CAD build for the part. Positions are in the model's coordinates, mm. A direction names the side the tool comes from. Round coordinates to 2 decimals unless told otherwise and drop trailing zeros. Loops run counter-clockwise (first coordinate to the right, second up) from the corner with the lowest first, then second, coordinate; pieces in that order, holes last. Notation, with made-up numbers: M 18.25,62 L 58.25,62 A30 ccw 58.25,91 Z; hole C -15.5,85 d7. An arc over 180 degrees is marked long. One line per item, written item: value. Start each with the question number.
from build123d import *

# Parameters (mm, degrees)
BASE_FLANGE1_DEPTH   = 0.7366
FILLET1_R            = 5
FILLET2_R            = 5
FILLET3_R            = 5
FILLET4_R            = 5
EDGE_FLANGE2_START   = -47.5
EDGE_FLANGE2_DEPTH   = 15.3683
EDGE_FLANGE2_START_2 = -32.5
EDGE_FLANGE2_2_DEPTH = 0.3683
EDGE_FLANGE2_3_DEPTH = 15
FILLET7_R            = 5
FILLET8_R            = 5
SKETCH18_R           = 1.5
CUT_EXTRUDE1_DEPTH   = 40
SKETCH23_R           = 1.52
CUT_EXTRUDE6_DEPTH   = 30
SKETCH24_R           = 1.52
CUT_EXTRUDE7_DEPTH   = 30
SKETCH25_R           = 1.4
CUT_EXTRUDE8_DEPTH   = 10


with BuildPart() as part:
    # Base-Flange1: sheet metal written as solids
    # Sketch1 → Base-Flange1 (new body)
    with BuildSketch(Plane(origin=(0, 0, 0), x_dir=(1, 0, 0), z_dir=(0, 1, 0))):
        Polygon((19.610938441, 32.5), (65, 32.5), (65, -32.5), (-65, -32.5), (-65, 32.5), (-19.610938441, 32.5), (-11.999061559, 32.5), (-11.999061559, 47.5), (12.000938441, 47.5), (12.000938441, 32.5), align=None)
    extrude(amount=-BASE_FLANGE1_DEPTH)

    # Fillet1
    fillet1_edges = [part.edges().sort_by_distance(p)[0] for p in [
        (65, -0.3683, 32.5),
    ]]
    fillet(fillet1_edges, radius=FILLET1_R)

    # Fillet2
    fillet2_edges = [part.edges().sort_by_distance(p)[0] for p in [
        (65, -0.3683, -32.5),
    ]]
    fillet(fillet2_edges, radius=FILLET2_R)

    # Fillet3
    fillet3_edges = [part.edges().sort_by_distance(p)[0] for p in [
        (-65, -0.3683, 32.5),
    ]]
    fillet(fillet3_edges, radius=FILLET3_R)

    # Fillet4
    fillet4_edges = [part.edges().sort_by_distance(p)[0] for p in [
        (-65, -0.3683, -32.5),
    ]]
    fillet(fillet4_edges, radius=FILLET4_R)

    # Edge-Flange2: read off the stored shape, not the designer's step
    # Edge-Flange2 outline → Edge-Flange2 (cut)
    with BuildSketch(Plane.XY.offset(EDGE_FLANGE2_START)):
        with BuildLine():
            ThreePointArc((-11.999061559, -0.197371375), (-11.643753776, -0.050198073), (-11.262461559, 0))
            Line((-11.262461559, 0), (-11.999061559, 0))
            Line((-11.999061559, 0), (-11.999061559, -0.197371375))
        make_face()
        with BuildLine():
            ThreePointArc((11.264338441, 0), (11.645630659, -0.050198073), (12.000938441, -0.197371375))
            Line((12.000938441, -0.197371375), (12.000938441, 0))
            Line((12.000938441, 0), (11.264338441, 0))
        make_face()
    extrude(amount=EDGE_FLANGE2_DEPTH, mode=Mode.SUBTRACT)

    # Edge-Flange2 2 outline → Edge-Flange2 2 (cut)
    with BuildSketch(Plane.XY.offset(EDGE_FLANGE2_START_2)):
        with BuildLine():
            Line((-11.999061559, -0.7366), (-10.894161559, -0.7366))
            Line((-10.894161559, -0.7366), (-10.894161559, 0))
            Line((-10.894161559, 0), (-11.262461559, 0))
            ThreePointArc((-11.262461559, 0), (-11.643753776, -0.050198073), (-11.999061559, -0.197371375))
            Line((-11.999061559, -0.197371375), (-11.999061559, -0.7366))
        make_face()
        with BuildLine():
            Line((12.000938441, -0.7366), (12.000938441, -0.197371375))
            ThreePointArc((12.000938441, -0.197371375), (11.645630659, -0.050198073), (11.264338441, 0))
            Line((11.264338441, 0), (10.896038441, 0))
            Line((10.896038441, 0), (10.896038441, -0.7366))
            Line((10.896038441, -0.7366), (12.000938441, -0.7366))
        make_face()
    extrude(amount=EDGE_FLANGE2_2_DEPTH, mode=Mode.SUBTRACT)

    # Edge-Flange2 3 outline → Edge-Flange2 3 (add)
    with BuildSketch(Plane.XY.offset(EDGE_FLANGE2_START)):
        with BuildLine():
            ThreePointArc((-11.999061559, -1.4732), (-11.783316414, -0.952345145), (-11.262461559, -0.7366))
            Line((-11.262461559, -0.7366), (-11.999061559, -0.7366))
            Line((-11.999061559, -0.7366), (-11.999061559, -0.197371375))
            ThreePointArc((-11.999061559, -0.197371375), (-12.538290183, -0.7366), (-12.735661559, -1.4732))
            Line((-12.735661559, -1.4732), (-12.735661559, -15))
            Line((-12.735661559, -15), (-11.999061559, -15))
            Line((-11.999061559, -15), (-11.999061559, -1.4732))
        make_face()
        with BuildLine():
            Line((12.737538441, -15), (12.737538441, -1.4732))
            ThreePointArc((12.737538441, -1.4732), (12.540167066, -0.7366), (12.000938441, -0.197371375))
            Line((12.000938441, -0.197371375), (12.000938441, -0.7366))
            Line((12.000938441, -0.7366), (11.264338441, -0.7366))
            ThreePointArc((11.264338441, -0.7366), (11.785193296, -0.952345145), (12.000938441, -1.4732))
            Line((12.000938441, -1.4732), (12.000938441, -15))
            Line((12.000938441, -15), (12.737538441, -15))
        make_face()
    extrude(amount=EDGE_FLANGE2_3_DEPTH)

    # Fillet7
    fillet7_edges = [part.edges().sort_by_distance(p)[0] for p in [
        (12.369238441, -15, -47.5),
    ]]
    fillet(fillet7_edges, radius=FILLET7_R)

    # Fillet8
    fillet8_edges = [part.edges().sort_by_distance(p)[0] for p in [
        (-12.367361559, -15, -47.5),
    ]]
    fillet(fillet8_edges, radius=FILLET8_R)

    # Sketch18 → Cut-Extrude1 (cut)
    with BuildSketch(Plane.ZY.offset(12.735661559)):
        with Locations(Location((-39.810498868, -4.68598948, 0), (0, 0, 270))):
            Circle(SKETCH18_R)
        with BuildLine():
            ThreePointArc((-39.496869826, -12.179429066), (-38.060907717, -10.61801534), (-39.622321443, -9.182053232))
            ThreePointArc((-39.622321443, -9.182053232), (-42.925238149, -7.933819403), (-44.310498868, -4.68598948))
            ThreePointArc((-44.310498868, -4.68598948), (-45.810498868, -3.18598948), (-47.310498868, -4.68598948))
            ThreePointArc((-47.310498868, -4.68598948), (-45.001731004, -10.099039351), (-39.496869826, -12.179429066))
        make_face()
    extrude(amount=-CUT_EXTRUDE1_DEPTH, mode=Mode.SUBTRACT)

    # Sketch23 → Cut-Extrude6 (cut)
    with BuildSketch(Plane(origin=(13.900294902, -97.850887802, -222.979867512), x_dir=(-3.678229639825758e-15, -0.0327435829113364, -0.9994637851258686), z_dir=(1, 0, 0))):
        with Locations(Location((-186.121703077, 87.117320509, 0), (0, 0, 271.876404504))):
            Circle(SKETCH23_R)
    extrude(amount=-CUT_EXTRUDE6_DEPTH, mode=Mode.SUBTRACT)

    # Sketch24 → Cut-Extrude7 (cut)
    with BuildSketch(Plane(origin=(13.900294902, -97.850887802, -222.979867512), x_dir=(-3.678229639825758e-15, -0.0327435829113364, -0.9994637851258686), z_dir=(1, 0, 0))):
        with Locations((-187.007062576, 81.183001798)):
            Circle(SKETCH24_R)
    extrude(amount=-CUT_EXTRUDE7_DEPTH, mode=Mode.SUBTRACT)

    # Sketch25 → Cut-Extrude8 (cut)
    with BuildSketch(Plane(origin=(-71.983966672, 0, -96.098250098), x_dir=(1, 0, 0), z_dir=(0, 1, 0))):
        with Locations(Location((79.090906604, -126.157708005, 0), (0, 0, 270))):
            Circle(SKETCH25_R)
        with Locations(Location((69.540906604, -126.157708005, 0), (0, 0, 270))):
            Circle(SKETCH25_R)
    extrude(amount=-CUT_EXTRUDE8_DEPTH, mode=Mode.SUBTRACT)


solid = part.part
(1) Flat gauge pins, fed straight in: P1, Ø5, axis at y = -10.59, z = -38.73, coming from the +X side; P2, Ø4, axis at x = -18, z = -9.5, coming from the -Y side; P3, Ø1.5, axis at y = -8.5, z = -38, coming from the -X side. Where does each tip first touch, or does it go through?
(2) Slice it at B-B, the plane z = 1. List the corners of the cut face in (x, y), and give its area (3 significant figures).
(3) Mould opens along Z. For faces 1 (the cylindrical face through (-63.57, -0.37, -31)), 2 (the cylindrical face through (63.57, -0.37, 31)), 3 (the cylindrical face through (-12.37, -10.04, -45.06)) say: pulls with the +Z half, pulls with the -Z half, needs draft (parallel to the pull), parting line crosses it, or undercut.
(4) Probe L1, parallel to Y at x = -32, z = 23.5; L2, parallel to X at y = -1.5, z = -41.5. List the from-to ranges inside material, lowest first.
(5) Which spindle directions (+Z, -Z, +X, -X, +Y, -Y) get a long thin tool onto all of the face, cutting with end or side? Do faces 4 (the flat face through (12.001, -8, -38)), 5 (the cylindrical face through (12.364, -7.969, -42.888)), 6 (the cylindrical face through (63.57, -0.37, -31)). Say none if no direction does.
(6) Slice it at A-A, the plane x = 34. List the corners of the cut face in (y, z), and give its area (3 significant figures).
Check result:
1. P1: stops at x = 12.74
1. P2: stops at y = -0.74
1. P3: stops at x = -12.74
2. outline: M -65,-0.74 L 65,-0.74 L 65,0 L -65,0 Z
2. area: 95.8 mm^2
3. face 1: pulls with the -Z half
3. face 2: pulls with the +Z half
3. face 3: undercut
4. L1: y = -0.74 to 0
4. L2: x = -12.74 to -12, 12 to 12.74
5. face 4: +Z, -Z, -Y
5. face 5: +X, -X
5. face 6: -Z, +X, +Y, -Y
6. outline: M -0.74,-32.5 L 0,-32.5 L 0,32.5 L -0.74,32.5 Z
6. area: 47.9 mm^2
